Source: CAD feature listing. Evaluate the final solid. Frame: model axes, mm. A direction names the side the tool comes from. Round coordinates to 2 decimals unless told otherwise and drop trailing zeros. Loops run counter-clockwise (first coordinate to the right, second up) from the corner with the lowest first, then second, coordinate; pieces in that order, holes last. Notation, with made-up numbers: M 55,31.25 L 98,31.25 A23 ccw 98,67.25 Z; hole C 56.25,86.25 d7. An arc over 180 degrees is marked long. One line per item, written item: value.
from build123d import *

# Parameters (mm, degrees)
CUT_EXTRUDE1_DEPTH = 9.525


with BuildPart() as part:
    # Sketch1 → Revolve1 (revolve)
    with BuildSketch(Plane.XY, mode=Mode.PRIVATE) as revolve1_sk:
        Polygon((0, 1.796034), (1.963185615, 1.27), (5.205360521, 1.27), (6.35, 3.175), (12.7, 3.175), (12.7, 5.5626), (38.1, 5.5626), (38.1, 12.7), (0, 12.7), align=None)
    revolve(revolve1_sk.sketch.rotate(Axis((0, 0, 0), (1, 0, 0)), 90), axis=Axis((0, 0, 0), (1, 0, 0)))

    # Sketch2 → Cut-Extrude1 (cut)
    with BuildSketch(Plane.ZY):
        with BuildLine():
            ThreePointArc((-9.525, 8.400260413), (-12.7, 0), (-9.525, -8.400260413))
            Line((-9.525, -8.400260413), (-9.525, 8.400260413))
        make_face()
        with BuildLine():
            Line((9.525, 8.400260413), (9.525, -8.400260413))
            ThreePointArc((9.525, -8.400260413), (11.879762203, -4.490128061), (12.7, 0))
            ThreePointArc((12.7, 0), (11.879762203, 4.490128061), (9.525, 8.400260413))
        make_face()
    extrude(amount=-CUT_EXTRUDE1_DEPTH, mode=Mode.SUBTRACT)


solid = part.part
1. Pin query (flat end, axial travel): pin 1 (10 mm diameter, centred on x = 17, y = -8.5, fed in from +Z); pin 2 (1 mm diameter, centred on x = 33.5, z = 4, fed in from +Y); pin 3 (3.5 mm diameter, centred on y = -1.5, z = 11.5, fed in from -X) (3 decimals). Return the tip coordinate at first contact, or that it passes through.
Report:
pin 1: stops at z = 12.21
pin 2: stops at y = 12.21
pin 3: stops at x = 9.525
2. Section query D-D (z = -4.5). Return the cut outline in (x, y).
Report:
outline: M 0,-11.88 L 38.1,-11.88 L 38.1,-3.27 L 12.7,-3.27 L 12.7,3.27 L 38.1,3.27 L 38.1,11.88 L 0,11.88 Z
3. Pull-direction query (Y, two-part tool) for faces 6 (the face through (18.783, -12.592, -1.653)), 7 (the face through (25.578, -1.671, 5.306)), 8 (the face through (9.57, 1.93, -2.52)), 9 (the face through (5, 0, 9.525)); classes: released by +Y, released by -Y, zero draft, split by the parting line, or undercut.
Report:
face 6: split by the parting line
face 7: undercut
face 8: undercut
face 9: zero draft
4. Ray query, line 1 (Y direction, x = 8.5, z = 0) (3 decimals); line 2 (Y direction, x = 2.9, z = 0); line 3 (X direction, y = 3.5, z = 0.75). Return the intervals inside material, ascending. Write a range as [from, to].
Report:
line 1: y = [-12.7, -3.175], [3.175, 12.7]
line 2: y = [-12.7, -1.27], [1.27, 12.7]
line 3: x = [0, 12.7]
5. Section query B-B (z = 0). Return the cut outline in (x, y) (3 decimals).
Report:
outline: M 0,-12.7 L 38.1,-12.7 L 38.1,-5.563 L 12.7,-5.563 L 12.7,-3.175 L 6.35,-3.175 L 5.205,-1.27 L 1.963,-1.27 L 0,-1.796 Z; M 0,1.796 L 1.963,1.27 L 5.205,1.27 L 6.35,3.175 L 12.7,3.175 L 12.7,5.563 L 38.1,5.563 L 38.1,12.7 L 0,12.7 Z
6. Section query C-C (x = 18). Return the cut outline in (y, z), and give its area (3 significant figures).
Report:
outline: C 0,0 d25.4; hole C 0,0 d11.13
area: 409 mm2
7. Reachability of faces 1 (the face through (5, 0, -9.525)), 2 (the face through (38.1, 3, -5)), 3 (the face through (12.7, 2.4, -2.4)), 4 (the face through (9.525, 0, 11)), 5 (the face through (1.432, 1.253, 0.652)) from +Z, -Z, +X, -X, +Y, -Y: full face, straight path, thin tool, end or side. Return the list, or none.
Report:
face 1: -Z, -X, +Y, -Y
face 2: +Z, -Z, +X, +Y, -Y
face 3: +X
face 4: +Z, -X, +Y, -Y
face 5: -X
8. Section query A-A (y = 0). Return the cut outline in (x, z) (3 decimals).
Report:
outline: M 0,-9.525 L 9.525,-9.525 L 9.525,-12.7 L 38.1,-12.7 L 38.1,-5.563 L 12.7,-5.563 L 12.7,-3.175 L 6.35,-3.175 L 5.205,-1.27 L 1.963,-1.27 L 0,-1.796 Z; M 0,1.796 L 1.963,1.27 L 5.205,1.27 L 6.35,3.175 L 12.7,3.175 L 12.7,5.563 L 38.1,5.563 L 38.1,12.7 L 9.525,12.7 L 9.525,9.525 L 0,9.525 Z
